Autodesk Inventor part; units mm, degrees
ref_plane "YZ Plane" through (0, 0, 0) normal (1, 0, 0) x (0, 1, 0)
ref_plane "XZ Plane" through (0, 0, 0) normal (0, 1, 0) x (-1, 0, 0)
ref_plane "XY Plane" through (0, 0, 0) normal (0, 0, 1) x (1, 0, 0)
sketch "Sketch1" plane through (0, 0, 0) normal (0, 0, 1) x (1, 0, 0)
  line L0 (-24.9, 24.9) -> (24.9, 24.9)
  line L1 (24.9, 24.9) -> (24.9, -24.9)
  line L2 (24.9, -24.9) -> (-24.9, -24.9)
  line L3 (-24.9, -24.9) -> (-24.9, 24.9)
  line L4 (-24.9, 24.9) -> (24.9, -24.9) construction
  line L5 (24.9, 24.9) -> (-24.9, -24.9) construction
  line L6 (17.05, 17.05) -> (-17.05, 17.05)
  line L7 (-17.05, 17.05) -> (-17.05, -17.05)
  line L8 (-17.05, -17.05) -> (17.05, -17.05)
  line L9 (17.05, -17.05) -> (17.05, 17.05)
  point P0 (0, 0)
  dimension "d0" = 49.8
  dimension "d1" = 49.8
  dimension "d2" = 7.85
extrude "Extrusion1" add sketch "Sketch1" along normal blind 7.7
sketch "Sketch2" plane through (0, 0, 7.7) normal (0, 0, 1) x (1, 0, 0)
  line L0 (17.05, 17.05) -> (17.05, -17.05)
  line L1 (17.05, -17.05) -> (-17.05, -17.05)
  line L2 (-17.05, -17.05) -> (-17.05, 17.05)
  line L3 (-17.05, 17.05) -> (17.05, 17.05)
  line L4 (24.9, 24.9) -> (-24.9, 24.9)
  line L5 (-24.9, 24.9) -> (-24.9, -24.9)
  line L6 (-24.9, -24.9) -> (24.9, -24.9)
  line L7 (24.9, -24.9) -> (24.9, 24.9)
  line L8 (17.05, -17.05) -> (24.9, -17.05)
  line L9 (24.9, -17.05) -> (24.9, -24.9)
  line L10 (24.9, -24.9) -> (17.05, -24.9)
  line L11 (17.05, -24.9) -> (17.05, -17.05)
  line L12 (17.05, 17.05) -> (-17.05, 17.05)
  line L13 (24.9, 24.9) -> (17.05, 24.9)
  line L14 (17.05, 24.9) -> (17.05, 17.05)
  line L15 (17.05, 17.05) -> (24.9, 17.05)
  line L16 (24.9, 17.05) -> (24.9, 24.9)
  line L17 (-24.9, -24.9) -> (-17.05, -24.9)
  line L18 (-17.05, -24.9) -> (-17.05, -17.05)
  line L19 (-17.05, -17.05) -> (-24.9, -17.05)
  line L20 (-24.9, -17.05) -> (-24.9, -24.9)
  line L21 (-24.9, 24.9) -> (-17.05, 24.9)
  line L22 (-17.05, 24.9) -> (-17.05, 17.05)
  line L23 (-17.05, 17.05) -> (-24.9, 17.05)
  line L24 (-24.9, 17.05) -> (-24.9, 24.9)
  point P0 (0, 0)
extrude "Extrusion2" add sketch "Sketch2" along normal blind 34.4 contours L14 L4 L7 L15 | L8 L7 L6 L11 | L23 L5 L4 L22 | L18 L6 L5 L19
sketch "Sketch3" plane through (0, 0, 0) normal (0, 0, -1) x (-1, 0, 0)
  line L0 (24.9, -24.9) -> (24.9, 24.9) construction
  line L1 (24.9, 24.9) -> (-24.9, 24.9) construction
  line L2 (-24.9, -24.9) -> (24.9, -24.9) construction
  line L3 (-24.9, 24.9) -> (-24.9, -24.9) construction
  point P0 (20, 20)
  point P1 (20, -20)
  point P2 (-20, -20)
  point P3 (-20, 20)
  dimension "d_1" = 4.9
  dimension "d96" = 4.9
  dimension "d97" = 4.9
  dimension "d98" = 4.9
  dimension "d99" = 4.9
  dimension "d100" = 4.9
  dimension "d101" = 4.9
  dimension "d102" = 4.9
hole "Hole1" at (-20, 20, 0) at (-20, -20, 0) at (20, -20, 0) at (20, 20, 0) direction (0, 0, 1) diameter 2.8 depth 16 counterbore diameter 5.5 counterbore depth 3.1
fillet "Fillet1" radius 2 8 edges at (24.9, 24.9, 21.05) (24.9, -24.9, 21.05) (-24.9, -24.9, 21.05) (-24.9, 24.9, 21.05) (-24.9, 0, 0) (0, -24.9, 0) (24.9, 0, 0) (0, 24.9, 0)
sketch "Sketch6" plane through (0, 0, 42.1) normal (0, 0, 1) x (1, 0, 0)
  arc A0 (-22.9, 24.9) -> (-24.9, 22.9) centre (-22.9, 22.9) ccw
  line L0 (-24.9, 22.9) -> (-24.9, 17.05)
  line L1 (-24.9, 17.05) -> (-17.05, 17.05)
  line L2 (-17.05, 17.05) -> (-17.05, 24.9)
  line L3 (-17.05, 24.9) -> (-22.9, 24.9)
  arc A1 (24.9, 22.9) -> (22.9, 24.9) centre (22.9, 22.9) ccw
  line L4 (22.9, 24.9) -> (17.05, 24.9)
  line L5 (17.05, 24.9) -> (17.05, 17.05)
  line L6 (17.05, 17.05) -> (24.9, 17.05)
  line L7 (24.9, 17.05) -> (24.9, 22.9)
  arc A2 (22.9, -24.9) -> (24.9, -22.9) centre (22.9, -22.9) ccw
  line L8 (24.9, -22.9) -> (24.9, -17.05)
  line L9 (24.9, -17.05) -> (17.05, -17.05)
  line L10 (17.05, -17.05) -> (17.05, -24.9)
  line L11 (17.05, -24.9) -> (22.9, -24.9)
  arc A3 (-24.9, -22.9) -> (-22.9, -24.9) centre (-22.9, -22.9) ccw
  line L12 (-22.9, -24.9) -> (-17.05, -24.9)
  line L13 (-17.05, -24.9) -> (-17.05, -17.05)
  line L14 (-17.05, -17.05) -> (-24.9, -17.05)
  line L15 (-24.9, -17.05) -> (-24.9, -22.9)
  line L16 (0, 38.1838) -> (54, 38.1838) construction
  line L17 (21.1338, 17.05) -> (17.05, 21.1338)
  line L18 (17.05, 24.9) -> (17.05, 17.05)
  line L19 (17.05, 21.1338) -> (17.05, 17.05)
  line L20 (17.05, 17.05) -> (21.1338, 17.05)
  line L21 (-17.05, 24.9) -> (-17.05, 17.05)
  line L22 (-17.05, 17.05) -> (-17.05, 21.1338)
  line L23 (-17.05, 21.1338) -> (-21.1338, 17.05)
  line L24 (-17.05, 21.1338) -> (-11.2747, 21.1338) construction
  line L25 (-17.05, -17.05) -> (-17.05, 17.05)
  line L26 (-21.1338, 17.05) -> (-17.05, 17.05)
  line L27 (-17.05, 17.05) -> (-21.1338, 17.05)
  line L28 (17.05, -17.05) -> (17.05, -24.9)
  line L29 (17.05, -17.05) -> (21.1338, -17.05)
  line L30 (24.9, -17.05) -> (17.05, -17.05)
  line L31 (21.1338, -17.05) -> (17.05, -21.1338)
  line L32 (17.05, -17.05) -> (17.05, -21.1338)
  line L33 (-17.05, -17.05) -> (-21.1338, -17.05)
  line L34 (-17.05, -17.05) -> (-17.05, -24.9)
  line L35 (-17.05, -17.05) -> (-17.05, -21.1338)
  line L36 (-21.1338, -17.05) -> (-17.05, -21.1338)
  line L37 (22.9, 22.9) -> (24.9, 22.9) construction
  line L38 (-22.9, -22.9) -> (22.9, 22.9) construction
  line L39 (-22.9, -22.9) -> (22.9, -22.9) construction
  line L40 (22.9, 22.9) -> (-22.9, 22.9) construction
  line L41 (22.9, -22.9) -> (-22.9, 22.9) construction
  dimension "d111" = 0
  dimension "d120" = 54
  dimension "d121" = 54
extrude "Extrusion3" cut sketch "Sketch6" against normal up to surface (34.4 mm away) contours L13 L36 L14 | L2 L1 L23 | L6 L5 L17 | L10 L9 L31
sketch "Sketch7" plane through (-24.9, 17.05, 7.7) normal (0, -1, 0) x (1, 0, 0)
  line L0 (41.95, 0) -> (49.95, 0) construction
  line L1 (41.95, -7.7) -> (41.95, 0) construction
  line L2 (7.85, -7.7) -> (7.85, 0) construction
  line L3 (-0.15, 0) -> (7.85, 0) construction
  line L4 (41.9235, 33.7204) -> (41.95, 0) construction
  line L5 (7.85, 0) -> (7.8764, 33.5861) construction
  line L6 (41.95, 0) -> (7.85, 0) construction
  circle A0 centre (24.9, 17.0366) radius 17.0366 construction
  line L7 (24.9, 55.2203) -> (-13.2838, 17.0366) construction
  line L8 (-13.2838, 17.0366) -> (24.9, -21.1472) construction
  line L9 (24.9, -21.1472) -> (63.0838, 17.0366) construction
  line L10 (63.0838, 17.0366) -> (24.9, 55.2203) construction
  line L11 (24.9, 55.2203) -> (24.9, -21.1472) construction
  line L12 (-13.2838, 17.0366) -> (63.0838, 17.0366) construction
  line L13 (24.9, 55.2203) -> (78.9, 55.2203) construction
  line L14 (46.1838, 0) -> (41.95, 0)
  line L15 (46.1838, 0) -> (41.95, -4.0972)
  line L16 (41.95, 0) -> (41.9235, 33.7204)
  line L17 (41.95, 0) -> (41.95, -4.0972)
  line L18 (46.1838, 0) -> (41.95, 0)
  line L19 (41.95, 0) -> (46.1838, 0)
  line L20 (7.85, 0) -> (3.6162, 0)
  line L21 (3.6162, 0) -> (7.85, -4.0972)
  line L22 (7.85, -4.0972) -> (7.85, 0)
  line L23 (24.9, -36.4773) -> (24.9, 70.8333)
  point P0 (44.386, 0)
  point P1 (43.5978, 0)
  point P2 (24.9, 17.0366)
  dimension "d37" = 54
  dimension "d38" = 135
  dimension "d39" = 54
extrude "Extrusion4" cut sketch "Sketch7" along normal up to surface (34.1 mm away)
sketch "Sketch8" plane through (17.05, -24.9, 7.7) normal (-1, 0, 0) x (0, 0, 1)
  line L0 (-4.0838, 41.95) -> (0, 41.95) construction
  line L1 (-4.0838, 7.85) -> (0.1503, 7.85) construction
  line L2 (0.1503, 7.85) -> (0.1503, 3.6159) construction
  line L3 (-4.0838, 7.85) -> (0.1503, 3.6159)
  line L4 (0.1503, 3.6159) -> (0.1503, 7.85)
  line L5 (0.1503, 7.85) -> (-4.0838, 7.85)
  line L6 (-4.0838, 41.95) -> (0, 46.0338)
  line L7 (-4.0838, 41.95) -> (1.6916, 41.95) construction
  line L8 (0.1503, 7.85) -> (0, 41.95)
  line L9 (0, 46.0338) -> (0, 41.95)
  line L10 (0, 41.95) -> (-4.0838, 41.95)
  line L11 (-6, 2) -> (-6, 47.8)
  line L12 (55.2338, 24.9) -> (17.05, 63.0838) construction
  line L13 (17.05, 63.0838) -> (-21.1338, 24.9) construction
  line L14 (-21.1338, 24.9) -> (17.05, -13.2838) construction
  line L15 (17.05, -13.2838) -> (55.2338, 24.9) construction
  line L16 (55.2338, 24.9) -> (-21.1338, 24.9) construction
  line L17 (17.05, 63.0838) -> (17.05, -13.2838) construction
  line L18 (-36.2573, 24.9) -> (70.6573, 24.9) construction
  line L19 (17.05, -28.5573) -> (17.05, 78.3573) construction
  line L20 (0, 41.95) -> (0, 43.5978) construction
  line L21 (0, 7.85) -> (-4.0972, 7.85) construction
  line L22 (-4.0972, 41.95) -> (-4.0972, 7.85) construction
  line L23 (0, 41.95) -> (-4.0972, 41.95) construction
  line L24 (0, 7.85) -> (0, 41.95) construction
  point P0 (-2.4341, 8)
  point P1 (0, 5.414)
  point P2 (17.05, 24.9)
  point P3 (17.05, 24.9)
  point P4 (17.05, 24.9)
  dimension "d122" = 54
  dimension "d123" = 54
extrude "Extrusion5" cut sketch "Sketch8" along normal up to surface (34.1 mm away)
sketch "Sketch9" plane through (0, 0, 42.1) normal (0, 0, 1) x (1, 0, 0)
  arc A0 (19.486, 18.6978) -> (18.6978, 19.486) centre (20, 20) ccw
  arc A1 (18.6978, -19.486) -> (19.486, -18.6978) centre (20, -20) ccw
  arc A2 (-19.486, -18.6978) -> (-18.6978, -19.486) centre (-20, -20) ccw
  arc A3 (-18.6978, 19.486) -> (-19.486, 18.6978) centre (-20, 20) ccw
hole "Hole2" at (20, 20, 42.1) at (-20, 20, 42.1) at (20, -20, 42.1) at (-20, -20, 42.1) direction (0, 0, -1) diameter 2.8 depth 12
sketch "Sketch15" plane through (0, 0, 0) normal (0, 0, -1) x (-1, 0, 0)
  line L0 (-17.05, -17.05) -> (-17.05, 17.05) construction
  line L1 (-17.05, 17.05) -> (17.05, 17.05) construction
  line L2 (17.05, 17.05) -> (17.05, -17.05) construction
  line L3 (17.05, -17.05) -> (-17.05, -17.05) construction
  circle A0 centre (-20, 20) radius 2.75 construction
  circle A1 centre (20, -20) radius 2.75 construction
  circle A2 centre (20, 20) radius 2.75 construction
  circle A3 centre (-20, -20) radius 2.75 construction
  line L4 (-22.9, 22.9) -> (22.9, 22.9) construction
  line L5 (-22.9, -22.9) -> (-22.9, 22.9) construction
  line L6 (22.9, -22.9) -> (-22.9, -22.9) construction
  line L7 (22.9, 22.9) -> (22.9, -22.9) construction
  line L8 (17.05, 21.1338) -> (-17.05, 21.1338) construction
  point P0 (0, 0)
  point P1 (-20.8, -14.5)
  point P2 (-14.5, -20.8)
  point P3 (14.5, -20.8)
  point P4 (20.8, -14.5)
  point P5 (20.8, 14.5)
  point P6 (14.5, 20.8)
  point P7 (-14.5, 20.8)
  point P8 (-20.8, 14.5)
hole "Hole8" at (14.5, -20.8, 0) at (20.8, -14.5, 0) at (-14.5, -20.8, 0) at (-20.8, -14.5, 0) at (-20.8, 14.5, 0) at (-14.5, 20.8, 0) at (14.5, 20.8, 0) at (20.8, 14.5, 0) direction (0, 0, 1) diameter 4.7 end through all
ref_plane "Arbeitsebene2" through (24.9, 0, 0) normal (-0.7071, 0, -0.7071) x (0, 1, 0)
ref_plane "Arbeitsebene3" through (0, -17.05, 7.7) normal (1, 0, 0) x (0, 0, -1)
ref_plane "Work Plane4" through (-17.05, 0, 7.7) normal (0, 1, 0) x (1, 0, 0)
equation "\"d1\" = d0"
equation "\"d121\" = d120"
properties part number "10_Cube_1x1_v3"
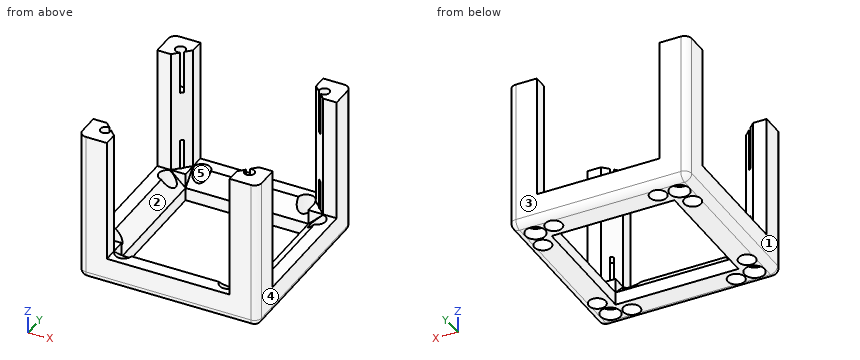
The listing builds one solid part. Answer for the finished solid, in the listing's coordinates (mm). Face numbers are marked on the shaded views. A direction names the side the tool comes from. Coordinates: 2 decimals unless noted, no trailing zeros. Write each loop counter-clockwise with the first axis right and the second up, starting at its lowest first coordinate (ties: lowest second). Pieces come first, ordered by that corner, then holes. Notation, with made-up numbers: (-16.5, 39.25) - (-5.5, 39.25) arc R31 ccw to (-5.5, 73.25) - close; hole circle Ø9 at (53.5, 80.5). An arc over 180 degrees is marked (long way). Return JSON: item names as keys, results as strings. Group by question number.
Q1. The part is cut by section B-B on z = 21.5. Write down the section's boundary in (x, y).
Q2. For a pull along Y with two mould halves and no side action, classify the marked faces 3, 4 and 5 as +Y half, -Y half, draft (parallel to the pull), parting line (faces both ways), or undercut.
Q3. The part is cut by section A-A on y = 11. Write down the section's boundary in (x, z).
Q4. Which of the six approach directions +Z, -Z, +X, -X, +Y, -Y give full straight-line access (tool end or side, diameter ignored) to the marked faces 1 and 2?
Q5. The part is cut by section C-C on x = 1. Write down the section's boundary in (y, z).
Q6. Flat-ended cylindrical pins translate along their axes: pin 1 Ø1.4 at (x, y) = (-20, -20.5) entering from -Z; pin 2 Ø4.5 at (x, y) = (20, 20) entering from -Z; pin 3 Ø3 at (x, y) = (6.5, 22.5) entering from +Z. Find the tip coordinate at first contact, or state that the pin passes through.
Q7. The part is cut by section D-D on x = 14.5. Write down the section's boundary in (y, z).
Q8. Find the intervals of material crossed by line 1 along Y through (x, z) = (4.5, 3.5); line 2 along X through (y, z) = (-14.5, 4.5); line 3 along Y through (x, z) = (20, 37), in increasing order. Write a range as [from, to].
Evaluation:
{
 "1": {"outline": "(-24.9, -22.9) arc R2 ccw to (-22.9, -24.9) - (-17.05, -24.9) - (-17.05, -21.13) - (-21.13, -17.05) - (-24.9, -17.05) - close; (-24.9, 17.05) - (-21.13, 17.05) - (-17.05, 21.13) - (-17.05, 24.9) - (-22.9, 24.9) arc R2 ccw to (-24.9, 22.9) - close; (17.05, -24.9) - (22.9, -24.9) arc R2 ccw to (24.9, -22.9) - (24.9, -17.05) - (21.13, -17.05) - (17.05, -21.13) - close; (17.05, 21.13) - (21.13, 17.05) - (24.9, 17.05) - (24.9, 22.9) arc R2 ccw to (22.9, 24.9) - (17.05, 24.9) - close"},
 "2": {"face 3": "+Y half", "face 4": "draft", "face 5": "undercut"},
 "3": {"outline": "(-24.9, 2) arc R2 ccw to (-22.9, 0) - (-17.05, 0) - (-17.05, 3.6) - (-21.28, 7.7) - (-24.9, 7.7) - close; (17.05, 0) - (22.9, 0) arc R2 ccw to (24.9, 2) - (24.9, 7.7) - (21.28, 7.7) - (17.05, 3.6) - close"},
 "4": {"face 1": "+Z, -Z, -X, +Y, -Y", "face 2": "+Z"},
 "5": {"outline": "(-24.9, 2) arc R2 ccw to (-22.9, 0) - (-17.05, 0) - (-17.05, 3.62) - (-21.13, 7.7) - (-24.9, 7.7) - close; (17.05, 0) - (22.9, 0) arc R2 ccw to (24.9, 2) - (24.9, 7.7) - (21.13, 7.7) - (17.05, 3.62) - close"},
 "6": {"pin 1": "stops at z = 16", "pin 2": "stops at z = 3.1", "pin 3": "stops at z = 7.7"},
 "7": {"outline": "(-24.9, 2) arc R2 ccw to (-23.15, 0.02) - (-23.15, 7.7) - (-24.9, 7.7) - close; (-18.45, 0) - (-17.05, 0) - (-17.05, 3.62) - (-18.45, 5.02) - close; (17.05, 0) - (18.45, 0) - (18.45, 5.02) - (17.05, 3.62) - close; (23.15, 0.02) arc R2 ccw to (24.9, 2) - (24.9, 7.7) - (23.15, 7.7) - close"},
 "8": {"line 1": "y = [-24.9, -17.05], [17.05, 24.9]", "line 2": "x = [-24.9, -23.15], [-18.45, -17.98], [17.98, 18.45], [23.15, 24.9]", "line 3": "y = [-24.9, -21.4], [-18.6, -18.18], [18.18, 18.6], [21.4, 24.9]"}
}
